```python
from build123d import *

# Parameters (mm, degrees)
SKETCH1_W           = 16
SKETCH1_H           = 16
SKETCH1_W_2         = 12
SKETCH1_H_2         = 12
BOSS_EXTRUDE1_DEPTH = 400
FILLET2_R           = 1
SKETCH2_R           = 2.5
CUT_EXTRUDE1_DEPTH  = 16


with BuildPart() as part:
    # Sketch1 → Boss-Extrude1 (new body)
    with BuildSketch(Plane(origin=(0, 0, 0), x_dir=(1, 0, 0), z_dir=(0, 1, 0))):
        with Locations((4.851851852, 0.925925926)):
            Rectangle(SKETCH1_W, SKETCH1_H)
        with Locations((4.851851852, 0.925925926)):
            Rectangle(SKETCH1_W_2, SKETCH1_H_2, mode=Mode.SUBTRACT)
    extrude(amount=BOSS_EXTRUDE1_DEPTH)

    # Fillet2
    fillet2_edges = [part.edges().sort_by_distance(p)[0] for p in [
        (-3.148148148, 200, -8.925925926),
        (12.851851852, 200, -8.925925926),
        (12.851851852, 200, 7.074074074),
        (-3.148148148, 200, 7.074074074),
    ]]
    fillet(fillet2_edges, radius=FILLET2_R)

    # Sketch2 → Cut-Extrude1 (cut)
    with BuildSketch(Plane.ZY.offset(3.148148148)):
        with Locations((-0.925925926, 8)):
            Circle(SKETCH2_R)
        with Locations((-0.925925926, 392)):
            Circle(SKETCH2_R)
    extrude(amount=-CUT_EXTRUDE1_DEPTH, mode=Mode.SUBTRACT)


solid = part.part
```
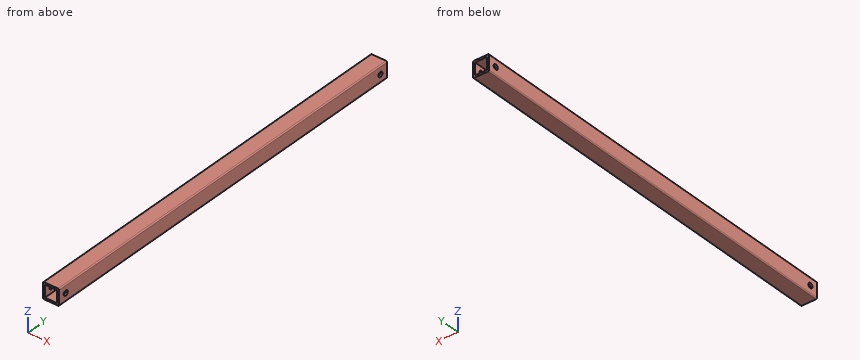
For this review, take the finished solid that the model builds, in its own axes (mm). Round coordinates to 2 decimals unless told otherwise and drop trailing zeros. Write each loop counter-clockwise with the first axis right and the second up, starting at its lowest first coordinate (ties: lowest second). Pieces come first, ordered by that corner, then holes. Notation, with made-up numbers: M -2,-20 L 14,-20 A28 cw 14,-2 Z; hole C 55.5,6 d10. An arc over 180 degrees is marked long. One line per item, written item: value. Start each with the question number.
(1) Insertion check: pin 1 (4 mm diameter, centred on y = 8, z = -0.93, fed in from +X). The pin has a flat end and moves straight along its axis. Give the tip position at first contact, or say it passes through.
(2) Wall thickness on line 1 (X direction, y = 321, z = 0.75); line 2 (Z direction, x = 11.95, y = 392); line 3 (Z direction, x = 2.5, y = 320): over which ranges is each line inside the solid? List them lowest first.
(3) We need section B-B (x = 5.25). Give the boundary of the cut face in (y, z), and give its area (3 significant figures).
(4) We need section A-A (y = 251.5). Give the boundary of the cut face in (x, z), and give its area (3 significant figures).
Result:
1. pin 1: through
2. line 1: -3.15 to -1.15, 10.85 to 12.85
2. line 2: -8.92 to -3.43, 1.57 to 7.07
2. line 3: -8.93 to -6.93, 5.07 to 7.07
3. outline: M 0,-8.93 L 400,-8.93 L 400,-6.93 L 0,-6.93 Z; M 0,5.07 L 400,5.07 L 400,7.07 L 0,7.07 Z
3. area: 1,600 mm²
4. outline: M -3.15,-7.93 A1 ccw -2.15,-8.93 L 11.85,-8.93 A1 ccw 12.85,-7.93 L 12.85,6.07 A1 ccw 11.85,7.07 L -2.15,7.07 A1 ccw -3.15,6.07 Z; hole M -1.15,-6.93 L 10.85,-6.93 L 10.85,5.07 L -1.15,5.07 Z
4. area: 111 mm²
